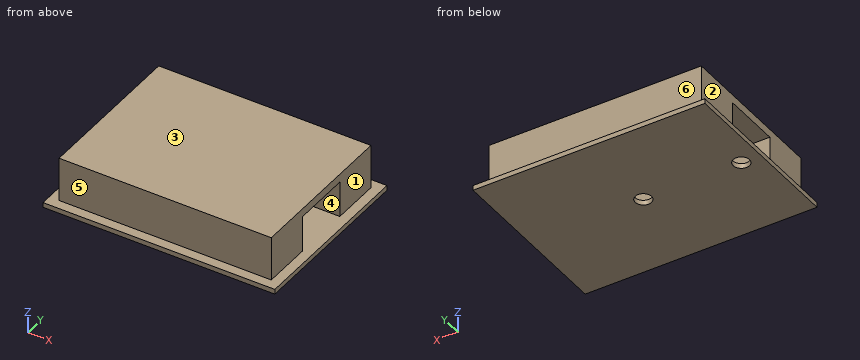
```python
from build123d import *

# Parameters (mm, degrees)
F0_W     = 71
F0_H     = 54
F1_DEPTH = 1.5
F2_R     = 2.5
F3_DEPTH = 25
F4_W     = 65
F4_H     = 15
F5_DEPTH = 11
F6_W     = 65
F6_H     = 48
F7_DEPTH = 2.5


with BuildPart() as f1:
    # F0 (on Top) → F1 (new body)
    with BuildSketch(Plane.XY):
        Rectangle(F0_W, F0_H)
    extrude(amount=F1_DEPTH)

    # F2 (on face) → F3 (cut)
    with BuildSketch(Plane.XY.offset(1.5)):
        with Locations((-29.5, 0)):
            Circle(F2_R)
        with Locations((0.5, 0)):
            Circle(F2_R)
    extrude(amount=-F3_DEPTH, mode=Mode.SUBTRACT)

    # F4 (on face) → F5 (join)
    with BuildSketch(Plane.XY.offset(1.5)):
        with Locations((0, 16.5)):
            Rectangle(F4_W, F4_H)
        with Locations((0, -16.5)):
            Rectangle(F4_W, F4_H)
    extrude(amount=F5_DEPTH)

    # F6 (on face) → F7 (join)
    with BuildSketch(Plane.XY.offset(12.5)):
        Rectangle(F6_W, F6_H)
    extrude(amount=F7_DEPTH)


solid = f1.part
```
Here's how the part is built. I have some questions about the finished solid (model axes, mm). Face numbers are marked on the shaded views. A direction names the side the tool comes from. Round coordinates to 2 decimals unless told otherwise and drop trailing zeros. Write each loop counter-clockwise with the first axis right and the second up, starting at its lowest first coordinate (ties: lowest second). Pieces come first, ordered by that corner, then holes.
Q1. If we section it at A-A on y = -5: Write out the boundary of the cut face in (x, z), plus the area to 3 significant figures.
Q2. If we section it at C-C on z = 5: Write out the boundary of the cut face in (x, y), plus the area to 3 significant figures.
Q3. If we mould it in two halves opening along Y, with no side actions, what happens to the marked faces 4, 5 and 6? For each: +Y half, -Y half, draft (parallel to the pull), parting line (faces both ways), or undercut.
Q4. If we section it at D-D on x = 0.5: Write out the boundary of the cut face in (y, z).
Q5. If we section it at B-B on x = 25: Write out the boundary of the cut face in (y, z).
Q6. Please list where these lines run through material, in increasing order: probe 1 along Y at (x, z) = (-1.5, 7.5); probe 2 along Y at (x, z) = (0.5, 1.1); probe 3 along X at (y, z) = (23.5, 7.25).
Q7. Which directions (+Z, -Z, +X, -X, +Y, -Y) give clear straight access to the entire face, cutting with the end or side of a thin tool? Please do the marked faces 1, 2 and 3.
Q8. Will these pins go through, and if not, where does the flat tip stop? P1, Ø4, axis at y = -17, z = 9.5, coming from the -X side; P2, Ø5.5, axis at x = 9.5, z = 7.5, coming from the +Y side; P3, Ø5.5, axis at x = -13, y = -2, coming from the -Z side; P4, Ø4.5, axis at x = -29.5, y = 0, coming from the -Z side.
Answer below:
1. outline: (-35.5, 0) - (35.5, 0) - (35.5, 1.5) - (-35.5, 1.5) - close; (-32.5, 12.5) - (32.5, 12.5) - (32.5, 15) - (-32.5, 15) - close
1. area: 269 mm2
2. outline: (-32.5, -24) - (32.5, -24) - (32.5, -9) - (-32.5, -9) - close; (-32.5, 9) - (32.5, 9) - (32.5, 24) - (-32.5, 24) - close
2. area: 1,950 mm2
3. face 4: undercut
3. face 5: -Y half
3. face 6: +Y half
4. outline: (-27, 0) - (-2.5, 0) - (-2.5, 1.5) - (-9, 1.5) - (-9, 12.5) - (9, 12.5) - (9, 1.5) - (2.5, 1.5) - (2.5, 0) - (27, 0) - (27, 1.5) - (24, 1.5) - (24, 15) - (-24, 15) - (-24, 1.5) - (-27, 1.5) - close
5. outline: (-27, 0) - (27, 0) - (27, 1.5) - (24, 1.5) - (24, 15) - (-24, 15) - (-24, 1.5) - (-27, 1.5) - close; hole (-9, 1.5) - (9, 1.5) - (9, 12.5) - (-9, 12.5) - close
6. probe 1: y = -24 to -9, 9 to 24
6. probe 2: y = -27 to -2.5, 2.5 to 27
6. probe 3: x = -32.5 to 32.5
7. face 1: +Z, +X, +Y, -Y
7. face 2: +Z, -X, +Y, -Y
7. face 3: +Z, +X, -X, +Y, -Y
8. P1: stops at x = -32.5
8. P2: stops at y = 24
8. P3: stops at z = 0
8. P4: stops at z = 12.5
